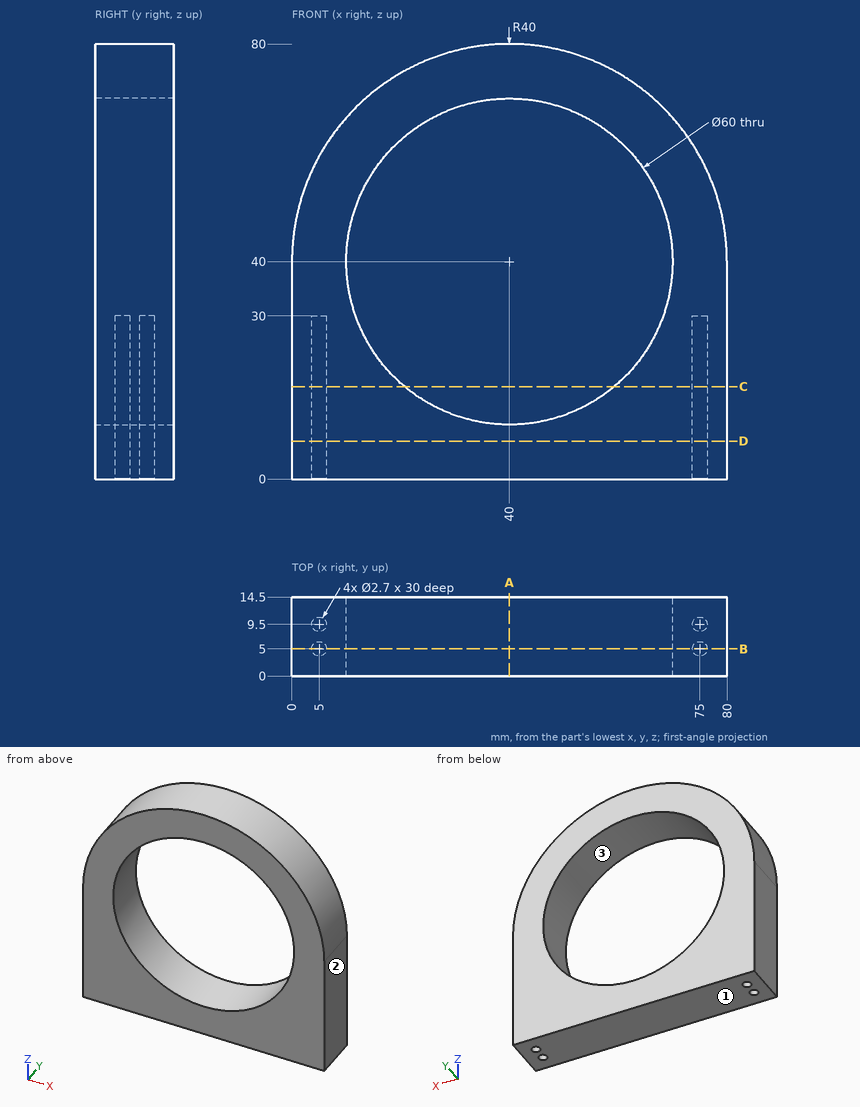
The drawing under review shows one solid part. Ordinate dimensions are in mm from its lowest x, y, z. Round coordinates to 2 decimals unless told otherwise and drop trailing zeros. Loops run counter-clockwise (first coordinate to the right, second up) from the corner with the lowest first, then second, coordinate; pieces in that order, holes last. Notation, with made-up numbers: (-10, 47.5) - (31, 47.5) arc R26 cw to (31, 74.5) - close; hole circle Ø3 at (-26.75, 48). An arc over 180 degrees is marked (long way). Put each result on its own line as item: value. Start each with the question number.
1. Consider section A-A on x = 40. State the section outline as (y, z) points.
2. Consider section D-D on z = 7. State the section outline as (x, y) points, plus the area to 3 significant figures.
3. Mouldability with a two-part tool opening along X and no side actions: class the marked faces 1, 2 and 3 as +X half, -X half, draft (parallel to the pull), parting line (faces both ways), or undercut.
4. Consider section C-C on z = 17. State the section outline as (x, y) points, plus the area to 3 significant figures.
5. Consider section B-B on y = 5. State the section outline as (x, z) points, plus the area to 3 significant figures.
6. For probe 1 along Y at (x, z) = (75, 19); probe 2 along X at (y, z) = (2.5, 39.5); probe 3 along Z at (x, y) = (30, 5.5), list the stretches that pass through material, from the lowest coordinate up. Write a range as [from, to].
7. Insertion check: P1, Ø6, axis at y = 3.5, z = 48.5, coming from the -X side; P2, Ø1, axis at x = 62, y = 1.5, coming from the -Z side; P3, Ø1.6, axis at x = 5, y = 5, coming from the -Z side; P4, Ø3, axis at y = 6.5, z = 66, coming from the +X side. Each pin has a flat end and moves straight along its axis. Give the tip position at first contact, or say it passes through.
Result sheet:
1. outline: (0, 0) - (14.5, 0) - (14.5, 10) - (0, 10) - close; (0, 70) - (14.5, 70) - (14.5, 80) - (0, 80) - close
2. outline: (0, 0) - (80, 0) - (80, 14.5) - (0, 14.5) - close; hole circle Ø2.7 at (5, 5); hole circle Ø2.7 at (5, 9.5); hole circle Ø2.7 at (75, 5); hole circle Ø2.7 at (75, 9.5)
2. area: 1,140 mm^2
3. face 1: draft
3. face 2: +X half
3. face 3: undercut
4. outline: (0, 0) - (20.74, 0) - (20.74, 14.5) - (0, 14.5) - close; (59.26, 0) - (80, 0) - (80, 14.5) - (59.26, 14.5) - close; hole circle Ø2.7 at (5, 5); hole circle Ø2.7 at (5, 9.5); hole circle Ø2.7 at (75, 5); hole circle Ø2.7 at (75, 9.5)
4. area: 579 mm^2
5. outline: (0, 0) - (3.65, 0) - (3.65, 30) - (6.35, 30) - (6.35, 0) - (73.65, 0) - (73.65, 30) - (76.35, 30) - (76.35, 0) - (80, 0) - (80, 40) arc R40 ccw to (0, 40) - close; hole circle Ø60 at (40, 40)
5. area: 2,720 mm^2
6. probe 1: [0, 3.65], [6.35, 8.15], [10.85, 14.5]
6. probe 2: [0, 10], [70, 80]
6. probe 3: [0, 11.72], [68.28, 78.73]
7. P1: x = 0.38
7. P2: z = 0
7. P3: z = 30
7. P4: x = 71.62
